```python
from build123d import *

# Parameters (mm, degrees)
SKETCH1_W           = 77.160601623
SKETCH1_H           = 44.898329167
BOSS_EXTRUDE1_DEPTH = 10
SKETCH2_R           = 11.353615653
CUT_EXTRUDE1_DEPTH  = 10


with BuildPart() as part:
    # Sketch1 → Boss-Extrude1 (new body)
    with BuildSketch(Plane(origin=(0, 0, 0), x_dir=(1, 0, 0), z_dir=(0, 1, 0))):
        with Locations((-16.668840769, 5.108193139)):
            Rectangle(SKETCH1_W, SKETCH1_H)
    extrude(amount=BOSS_EXTRUDE1_DEPTH)

    # Sketch2 → Cut-Extrude1 (cut)
    with BuildSketch(Plane(origin=(0, 10, 0), x_dir=(1, 0, 0), z_dir=(0, 1, 0))):
        with Locations((-30.666389333, 9.777294834)):
            Circle(SKETCH2_R)
    extrude(amount=-CUT_EXTRUDE1_DEPTH, mode=Mode.SUBTRACT)


solid = part.part
```
CAD build for the part. Positions are in the model's coordinates, mm. Give positions to 0.01 mm unless a question says otherwise; leave off trailing zeros. Order: outer loops, then holes, each group sorted by start corner. A loop starts at its lowest first (then second) coordinate and runs counter-clockwise, first axis right, second up.
(1) Drill centre lines: L1, parallel to X at y = 9, z = -10; L2, parallel to X at y = 8.5, z = -14.5; L3, parallel to Z at x = -28.5, y = 4.5. Where is each one in solid material? Low to high.
(2) Saw through at B-B, the plane z = -20. Give the cut face in (x, y).
(3) Saw through at C-C, the plane y = 8.25. Give the cut face in (x, z).
(4) Saw through at A-A, the plane x = -30. Give the cut face in (y, z).
(5) Mould opens along X. For faces 1 (the flat face through (-55.249, 5, -5)), 2 (the flat face through (-17, 5, 17.341)), 3 (the flat face through (21.911, 5, -5)), 4 (the cylindrical face through (-42.01, 5.07, -10.28)) say: released by +X, released by -X, zero draft, split by the parting line, or undercut.
Results found:
1. L1: x = -55.25 to -42.02, -19.31 to 21.91
1. L2: x = -55.25 to -40.99, -20.34 to 21.91
1. L3: z = -27.56 to -20.92, 1.37 to 17.34
2. outline: (-55.25, 0) - (-35.61, 0) - (-35.61, 10) - (-55.25, 10) - close; (-25.73, 0) - (21.91, 0) - (21.91, 10) - (-25.73, 10) - close
3. outline: (-55.25, -27.56) - (21.91, -27.56) - (21.91, 17.34) - (-55.25, 17.34) - close; hole circle Ø22.71 at (-30.67, -9.78)
4. outline: (0, -27.56) - (10, -27.56) - (10, -21.11) - (0, -21.11) - close; (0, 1.56) - (10, 1.56) - (10, 17.34) - (0, 17.34) - close
5. face 1: released by -X
5. face 2: zero draft
5. face 3: released by +X
5. face 4: undercut
